from build123d import *

# Parameters (mm, degrees)
BOSS_EXTRUDE1_DEPTH = 0.65
SKETCH2_W           = 0.65
SKETCH2_H           = 9.465837675
CUT_EXTRUDE1_DEPTH  = 12.29
BOSS_EXTRUDE2_DEPTH = 0.35
BOSS_EXTRUDE3_DEPTH = 0.96
BOSS_EXTRUDE4_DEPTH = 0.96
DRAFT1_START        = 1.31
DRAFT1_DEPTH        = 0.65
DRAFT2_DEPTH        = 1.96
DRAFT2_START        = 1.31
DRAFT2_2_DEPTH      = 0.65
HOLE1_D             = 1.3
HOLE1_CBORE_D       = 2.5
HOLE1_CBORE_DEPTH   = 0.96
HOLE2_D             = 2
HOLE2_DEPTH         = 1.960025
HOLE2_CSINK_D       = 2.7
HOLE2_CSINK_ANGLE   = 90
HOLE3_D             = 1.8
HOLE3_DEPTH         = 1.960025
HOLE3_CSINK_D       = 2.4
HOLE3_CSINK_ANGLE   = 90
CHAMFER1_SIZE       = 0.25
FILLET1_R           = 0.25
FILLET2_R           = 4.6


# Read off the part's stored shape, not the designer's step: Draft1, Draft2
with BuildPart() as part:
    # Sketch1 → Boss-Extrude1 (new body)
    with BuildSketch(Plane.XY.offset(1.96)):
        with BuildLine():
            Line((-3.74, -3.59), (-12.32, -13.328169417))
            ThreePointArc((-12.32, -13.328169417), (-0.020405468, -18.149988529), (12.29, -13.355837675))
            Line((12.29, -13.355837675), (12.29, -3.59))
            Line((12.29, -3.59), (-3.74, -3.59))
        make_face()
    extrude(amount=-BOSS_EXTRUDE1_DEPTH)

    # Sketch2 → Cut-Extrude1 (cut)
    with BuildSketch(Plane(origin=(12.29, 0, 0), x_dir=(0, 0, -1), z_dir=(1, 0, 0))):
        with Locations((-1.635, -8.322918838)):
            Rectangle(SKETCH2_W, SKETCH2_H)
    extrude(amount=-CUT_EXTRUDE1_DEPTH, mode=Mode.SUBTRACT)

    # Sketch3 → Boss-Extrude2 (add)
    with BuildSketch(Plane(origin=(0, 0, 1.31), x_dir=(-1, 0, 0), z_dir=(0, 0, -1))):
        with BuildLine():
            Line((1.143818798, -15.746447607), (8.016709975, -8.444000732))
            Line((8.016709975, -8.444000732), (12.32, -13.328169417))
            ThreePointArc((12.32, -13.328169417), (0.020405468, -18.149988529), (-12.29, -13.355837675))
            Line((-12.29, -13.355837675), (-12.29, -13.055837675))
            Line((-12.29, -13.055837675), (-5.126410253, -13.055837675))
            Line((-5.126410253, -13.055837675), (1.143818798, -15.746447607))
        make_face()
    extrude(amount=BOSS_EXTRUDE2_DEPTH)

    # Sketch4 → Boss-Extrude3 (add)
    with BuildSketch(Plane(origin=(0, 0, 0.96), x_dir=(-1, 0, 0), z_dir=(0, 0, -1))):
        with BuildLine():
            Line((-12.29, -13.055837675), (-5.126410253, -13.055837675))
            Line((-5.126410253, -13.055837675), (-3.369826358, -13.809603133))
            ThreePointArc((-3.369826358, -13.809603133), (-3.436718106, -15.84520854), (-4.497267699, -17.584000775))
            ThreePointArc((-4.497267699, -17.584000775), (-8.655774373, -15.953058328), (-12.29, -13.355837675))
            Line((-12.29, -13.355837675), (-12.29, -13.055837675))
        make_face()
    extrude(amount=BOSS_EXTRUDE3_DEPTH)

    # Sketch5 → Boss-Extrude4 (add)
    with BuildSketch(Plane(origin=(0, 0, 0.96), x_dir=(-1, 0, 0), z_dir=(0, 0, -1))):
        with BuildLine():
            Line((4.563917341, -12.112592905), (8.016709975, -8.444000732))
            Line((8.016709975, -8.444000732), (12.32, -13.328169417))
            ThreePointArc((12.32, -13.328169417), (9.811348174, -15.269575862), (7.003003277, -16.744564644))
            ThreePointArc((7.003003277, -16.744564644), (4.920508914, -14.882988414), (4.563917341, -12.112592905))
        make_face()
    extrude(amount=BOSS_EXTRUDE4_DEPTH)

    # Draft1 outline → Draft1 (add)
    with BuildSketch(Plane.XY.offset(DRAFT1_START)):
        Polygon((0, -13.055837675), (8.909023694, -13.055837675), (0, -3.59), align=None)
    extrude(amount=DRAFT1_DEPTH)

    # Draft2 outline → Draft2 (add)
    with BuildSketch(Plane.XY):
        Polygon((12.29, -13.055837675), (9.025, -11.382918837), (5.126410253, -13.055837675), align=None)
    extrude(amount=DRAFT2_DEPTH)

    # Draft2 2 outline → Draft2 2 (add)
    with BuildSketch(Plane.XY.offset(DRAFT2_START)):
        Polygon((7.820834561, -11.899636721), (9.025, -11.382918837), (5.76, -9.71), align=None)
    extrude(amount=DRAFT2_2_DEPTH)

    # Hole1 (through all)
    with Locations(Plane.XY.offset(1.96)):
        with Locations((7.269383833, -14.700362078), (-8.459801911, -13.019281065)):
            CounterBoreHole(HOLE1_D / 2, HOLE1_CBORE_D / 2, HOLE1_CBORE_DEPTH)

    # Hole2
    with Locations(Plane.XY.offset(1.96)):
        with Locations((0, -10.25), (-2.662261998, -6.0740848)):
            CounterSinkHole(HOLE2_D / 2, HOLE2_CSINK_D / 2, depth=HOLE2_DEPTH, counter_sink_angle=HOLE2_CSINK_ANGLE)

    # Hole3
    with Locations(Plane.XY.offset(1.96)):
        with Locations((4.697017702, -10.646000252)):
            CounterSinkHole(HOLE3_D / 2, HOLE3_CSINK_D / 2, depth=HOLE3_DEPTH, counter_sink_angle=HOLE3_CSINK_ANGLE)

    # Chamfer1
    chamfer1_edges = [part.edges().sort_by_distance(p)[0] for p in [
        (-9.709801911, -13.019281065, 1.96),
        (6.019383833, -14.700362078, 1.96),
    ]]
    chamfer(chamfer1_edges, length=CHAMFER1_SIZE)

    # Fillet1
    fillet1_edges = [part.edges().sort_by_distance(p)[0] for p in [
        (5.76, -9.71, 1.635),
        (-12.32, -13.328169417, 0.98),
        (12.29, -13.055837675, 0.98),
        (12.29, -13.355837675, 0.98),
        (0, -3.59, 1.635),
        (-3.74, -3.59, 1.635),
    ]]
    fillet(fillet1_edges, radius=FILLET1_R)

    # Fillet2
    fillet2_edges = [part.edges().sort_by_distance(p)[0] for p in [
        (-1.143818798, -15.746447607, 1.135),
    ]]
    fillet(fillet2_edges, radius=FILLET2_R)


solid = part.part
The model under review builds one solid part; all positions refer to its coordinate system, in mm. A direction names the side the tool comes from. Round coordinates to 2 decimals unless told otherwise and drop trailing zeros. Loops run counter-clockwise (first coordinate to the right, second up) from the corner with the lowest first, then second, coordinate; pieces in that order, holes last. Notation, with made-up numbers: (80.5, -17) -> (133.5, -17) arc R16 cw to (133.5, 13) -> close; hole circle Ø9 at (11, 85.5). An arc over 180 degrees is marked (long way). Write item = value, one per line. Start each with the question number.
Item 1: Insertion check: pin 1 (1.5 mm diameter, centred on x = -8.46, y = -13.02, fed in from +Z); pin 2 (2.5 mm diameter, centred on x = 0, y = -10.25, fed in from -Z); pin 3 (5 mm diameter, centred on x = -0.5, y = -16, fed in from -Z). Each pin has a flat end and moves straight along its axis. Give the tip position at first contact, or say it passes through.
Item 2: Take a section at C-C on y = -10.25. Count the separate pieces of the cut face and the enclosed holes in it, plus the area to 3 significant figures.
Item 3: To check wall thickness, follow L1, parallel to X at y = -10.25, z = 1.55; L2, parallel to X at y = -14, z = 1.5; L3, parallel to X at y = -16, z = 0.15. State the ranges of each line that lie inside material, in increasing order.
Item 4: For faces 1 (the cylindrical face through (3.43, -15.82, 0.49)), 2 (the cylindrical face through (7, -15.92, 1.36)), 3 (the flat face through (-7.5, -13.5, 0)), 4 (the flat face through (-2, -9, 1.31)), list the 3-axis set-ups (+Z, -Z, +X, -X, +Y, -Y) from which the entire face can be reached by the end or side of a thin tool; tool diameter is ignored.
Item 5: Take a section at A-A on z = 0.5. Give the boundary of the cut face in (x, y) (3 decimals).
Item 6: Mouldability with a two-part tool opening along Y and no side actions: class faces 5 (the cylindrical face through (-0.9, -14.76, 1.13)), 6 (the flat face through (0, -12, 1.96)), 7 (the cylindrical face through (-8.375, -12.375, 0.493)) as released by +Y, released by -Y, zero draft, split by the parting line, or undercut.
Item 7: Take a section at B-B on y = -16.5. Give the boundary of the cut face in (x, z), plus the area to 3 significant figures.
Result:
q1.pin_1 = 1
q1.pin_2 = 1.31
q1.pin_3 = 0.96
q2.separate_pieces = 3
q2.enclosed_holes = 0
q2.area = 12.4 mm²
q3.L1 = -9.61 to -1, 1 to 3.89, 5.51 to 6.81
q3.L2 = -11.55 to -9.23, -7.68 to 6.23, 8.3 to 11.55
q3.L3 = -8.57 to -5.79, 3.49 to 8.57
q4.face_1 = -Z
q4.face_2 = +Z
q4.face_3 = -Z, +X, -X, +Y, -Y
q4.face_4 = -Z, +Y
q5.outline = (-12.158, -13.144) arc R0.25 ccw to (-12.137, -13.495) arc R18.15 ccw to (-7.003, -16.745) arc R4 ccw to (-4.564, -12.113) -> (-8.017, -8.444) -> close; (3.37, -13.81) arc R4 ccw to (4.497, -17.584) arc R18.15 ccw to (12.208, -13.431) arc R0.25 ccw to (12.29, -13.246) -> (12.29, -13.209) arc R0.25 ccw to (12.154, -12.986) -> (9.025, -11.383) -> close; hole circle Ø1.3 at (-8.46, -13.019); hole circle Ø1.3 at (7.269, -14.7)
q6.face_5 = released by +Y
q6.face_6 = zero draft
q6.face_7 = undercut
q7.outline = (-7.56, 0) -> (-6.49, 0) -> (-6.49, 0.96) -> (3.7, 0.96) -> (3.7, 0) -> (7.56, 0) -> (7.56, 1.96) -> (-7.56, 1.96) -> close
q7.area = 19.9 mm²
